Answer from the drawing. Dimensions are ordinates in mm from the lowest x, y and z of the part. A direction names the side the tool comes from. Round coordinates to 2 decimals unless told otherwise and drop trailing zeros. Write each loop counter-clockwise with the first axis right and the second up, starting at its lowest first coordinate (ties: lowest second). Pieces come first, ordered by that corner, then holes. Notation, with made-up numbers: M -32,-20 L -11,-20 A18 cw -11,11 Z; hole C -5.5,0 d1. An arc over 180 degrees is marked long. Answer as CSV lines item,"result". Start each with the question number.
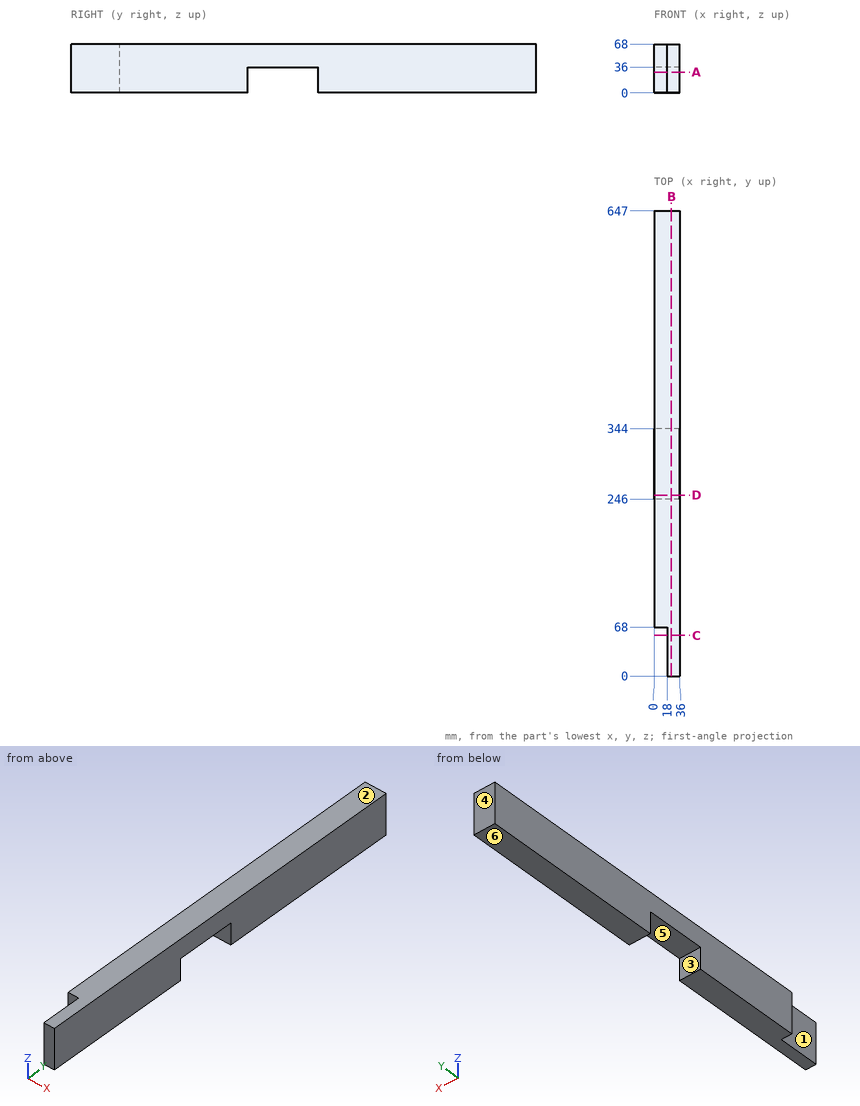
Q1. The mould has two halves that part along Y. Classify the marked faces 3, 4, 5 and 6: +Y half, -Y half, draft (parallel to the pull), parting line (faces both ways), or undercut.
Q2. Find section C-C (y = 56.5). Determine the outline of the cut face in (x, z).
Q3. Straight lines are drawn through the part: L1, parallel to Y at x = 24, z = 28.5; L2, parallel to Y at x = 2, z = 14.5; L3, parallel to Y at x = 3, z = 49. For each, find the intervals that lie inside material, in ascending order.
Q4. Find section B-B (x = 24). Determine the outline of the cut face in (y, z), plus the area to 3 significant figures.
Q5. Find section D-D (y = 251.5). Determine the outline of the cut face in (x, z).
Q6. Find section A-A (z = 29). Determine the outline of the cut face in (x, y), plus the area to 3 significant figures.
Q7. Each of these flat-tipped pins is pushed along its axis until it touches: P1, Ø12, axis at x = 10, y = 150.5, coming from the -Z side; P2, Ø18, axis at x = 14.5, y = 314.5, coming from the -Z side; P3, Ø14.5, axis at x = 6.5, z = 21.5, coming from the -Y side. Where does it stop, or does it pass through?
Q8. For the marked faces 1 and 2, determine the directions among +Z, -Z, +X, -X, +Y, -Y from which every point of the face is accessible in a straight line to the end or side of a thin tool.
Reported:
1,face 3,"undercut"
1,face 4,"+Y half"
1,face 5,"undercut"
1,face 6,"draft"
2,outline,"M 18,0 L 36,0 L 36,68 L 18,68 Z"
3,L1,"y = 0 to 246, 344 to 647"
3,L2,"y = 68 to 246, 344 to 647"
3,L3,"y = 68 to 647"
4,outline,"M 0,0 L 246,0 L 246,36 L 344,36 L 344,0 L 647,0 L 647,68 L 0,68 Z"
4,area,"40,500 mm2"
5,outline,"M 0,36 L 36,36 L 36,68 L 0,68 Z"
6,outline,"M 0,68 L 18,68 L 18,0 L 36,0 L 36,246 L 0,246 Z; M 0,344 L 36,344 L 36,647 L 0,647 Z"
6,area,"18,500 mm2"
7,P1,"stops at z = 0"
7,P2,"stops at z = 36"
7,P3,"stops at y = 68"
8,face 1,"+Z, -Z, -X, -Y"
8,face 2,"+Z, +X, -X, +Y, -Y"
